```python
from build123d import *

# Parameters (mm, degrees)
F1_DEPTH = 50
F2_DEPTH = 3
F4_DEPTH = 103


with BuildPart() as f1:
    # F0 (on Top) → F1 (new body)
    with BuildSketch(Plane.XY):
        with BuildLine():
            Line((-51.5, 0), (-48.5, 0))
            Line((-48.5, 0), (-48.5, 95))
            ThreePointArc((-48.5, 95), (-47.0355339059, 98.5355339059), (-43.5, 100))
            Line((-43.5, 100), (43.5, 100))
            ThreePointArc((43.5, 100), (47.0355339059, 98.5355339059), (48.5, 95))
            Line((48.5, 95), (48.5, 0))
            Line((48.5, 0), (51.5, 0))
            Line((51.5, 0), (51.5, 95))
            ThreePointArc((51.5, 95), (49.1568542495, 100.6568542495), (43.5, 103))
            Line((43.5, 103), (-43.5, 103))
            ThreePointArc((-43.5, 103), (-49.1568542495, 100.6568542495), (-51.5, 95))
            Line((-51.5, 95), (-51.5, 0))
        make_face()
    extrude(amount=F1_DEPTH)

    # F0 (on Top) → F2 (join)
    with BuildSketch(Plane.XY):
        with BuildLine():
            Line((-58.5, 0), (-51.5, 0))
            Line((-51.5, 0), (-51.5, 95))
            ThreePointArc((-51.5, 95), (-49.1568542495, 100.6568542495), (-43.5, 103))
            Line((-43.5, 103), (43.5, 103))
            ThreePointArc((43.5, 103), (49.1568542495, 100.6568542495), (51.5, 95))
            Line((51.5, 95), (51.5, 0))
            Line((51.5, 0), (58.5, 0))
            Line((58.5, 0), (58.5, 95))
            ThreePointArc((58.5, 95), (54.1066017178, 105.6066017178), (43.5, 110))
            Line((43.5, 110), (-43.5, 110))
            ThreePointArc((-43.5, 110), (-54.1066017178, 105.6066017178), (-58.5, 95))
            Line((-58.5, 95), (-58.5, 0))
        make_face()
    extrude(amount=F2_DEPTH)

    # F3 (on face) → F4 (cut, through all)
    with BuildSketch(Plane(origin=(-51.5, 0, 0), x_dir=(0, -1, 0), z_dir=(-1, 0, 0))):
        with BuildLine():
            Line((0, 50), (-95, 50))
            add(Edge.make_bspline(
                [(-95, 50), (-31.6906612889, 50), (-12.9379844293, 4.3437238783), (0, 3)],
                knots=[0, 0, 0, 0, 105.9905656179, 105.9905656179, 105.9905656179, 105.9905656179], degree=3))
            Line((0, 3), (0, 50))
        make_face()
    extrude(amount=-F4_DEPTH, mode=Mode.SUBTRACT)


solid = f1.part
```
Geometry check sheet. Reference: the model listing, model coordinates, mm. A direction names the side the tool comes from. Round coordinates to 2 decimals unless told otherwise and drop trailing zeros. Loops run counter-clockwise (first coordinate to the right, second up) from the corner with the lowest first, then second, coordinate; pieces in that order, holes last. Notation, with made-up numbers: (1, -25) - (53, -25) arc R15 ccw to (53, -10) - close; hole circle Ø1 at (80, 39.25). An arc over 180 degrees is marked (long way). Write each question's results on one line, items separated by ' | '. Start each with the question number.
Q1. Gauge pin test, flat ends, axial feed: P1, Ø14, axis at x = 4.5, z = 25.5, coming from the +Y side; P2, Ø3, axis at x = -39.5, z = 35.5, coming from the -Y side; P3, Ø14, axis at y = 55, z = 27.5, coming from the +X side. Record the tip position at first contact, or that the pin passes through.
Q2. Cross-section at A-A on x = -6.5. Enter the section's corners in (y, z), and give its area (3 significant figures).
Q3. Thickness scan on line 1 (X direction, y = 72, z = 38.5); line 2 (Y direction, x = 19.5, z = 38); line 3 (Y direction, x = 47, z = 39.5). Record the ranges inside material, lowest first. Write a range as [from, to].
Q4. Cross-section at B-B on y = 98. Enter the section's corners in (x, z).
Q5. Access from +Z, -Z, +X, -X, +Y, -Y to the whole of each face (thin tool, end or side, straight path). Record for faces 5 (the cylindrical face through (-49.094, 100.719, 26.171)), 6 (the cylindrical face through (47, 98.57, 24.65)), 7 (the flat face through (-5, 104, 3)), 8 (the flat face through (1, 103, 26)).
Q6. Cross-section at C-C on x = -45. Enter the section's corners in (y, z), and give its area (3 significant figures).
Q7. Release check for a two-part mould opening along X. For faces 1 (the flat face through (-1, 100, 25)), 2 (the cylindrical face through (49.219, 100.594, 26.171)), 3 (the flat face through (0, 104, 0)), 4 (the cylindrical face through (-53.99, 105.72, 1.48)) record: +X half, -X half, draft (parallel to the pull), parting line (faces both ways), or undercut.
Answers below:
1) P1: stops at y = 103 | P2: stops at y = 100 | P3: stops at x = 51.5
2) outline: (100, 0) - (110, 0) - (110, 3) - (103, 3) - (103, 50) - (100, 50) - close | area: 171 mm²
3) line 1: x = [-51.5, -48.5], [48.5, 51.5] | line 2: y = [100, 103] | line 3: y = [98.57, 102.19]
4) outline: (-58.2, 0) - (-47.5, 0) - (-47.5, 50) - (-50.92, 50) - (-50.92, 3) - (-58.2, 3) - close; (47.5, 0) - (58.2, 0) - (58.2, 3) - (50.92, 3) - (50.92, 50) - (47.5, 50) - close
5) face 5: +Z, -X, +Y | face 6: +Z, -Z, -Y | face 7: +Z, +Y | face 8: +Z, +X, -X, +Y
6) outline: (99.77, 0) - (109.92, 0) - (109.92, 3) - (102.86, 3) - (102.86, 50) - (99.77, 50) - close | area: 176 mm²
7) face 1: undercut | face 2: +X half | face 3: draft | face 4: -X half
